Part print with two shaded views. Sizes in mm from the minimum x, y, z corner. Give positions to 0.01 mm unless a question says otherwise; leave off trailing zeros. Order: outer loops, then holes, each group sorted by start corner. A loop starts at its lowest first (then second) coordinate and runs counter-clockwise, first axis right, second up. Notation, with made-up numbers: (81, -36) -> (94, -36) arc R6 ccw to (94, -31) -> close; hole circle Ø4 at (38, -13). An arc over 180 degrees is marked (long way). Write item = value, one per line. Start each with the question number.
Item 1: Flat gauge pins, fed straight in: P1, Ø3, axis at x = 11.5, z = 11.5, coming from the +Y side; P2, Ø12, axis at x = 176, z = 55.5, coming from the +Y side. Where does each tip first touch, or does it go through?
Item 2: Band-saw the part on B-B on x = 111.5. Write the cut outline in (y, z).
Item 3: Band-saw the part on D-D on x = 76.5. Write the cut outline in (y, z), plus the area to 3 significant figures.
Item 4: Drill centre lines: line 1 along X through (y, z) = (3.75, 11.5); line 2 along Z through (x, y) = (211.5, 7); line 3 along X through (y, z) = (1, 12.5). Where is each one in solid material? Low to high.
Item 5: Band-saw the part on A-A on z = 86.5. Write the cut outline in (x, y).
Item 6: Band-saw the part on C-C on z = 18.5. Write the cut outline in (x, y), plus the area to 3 significant figures.
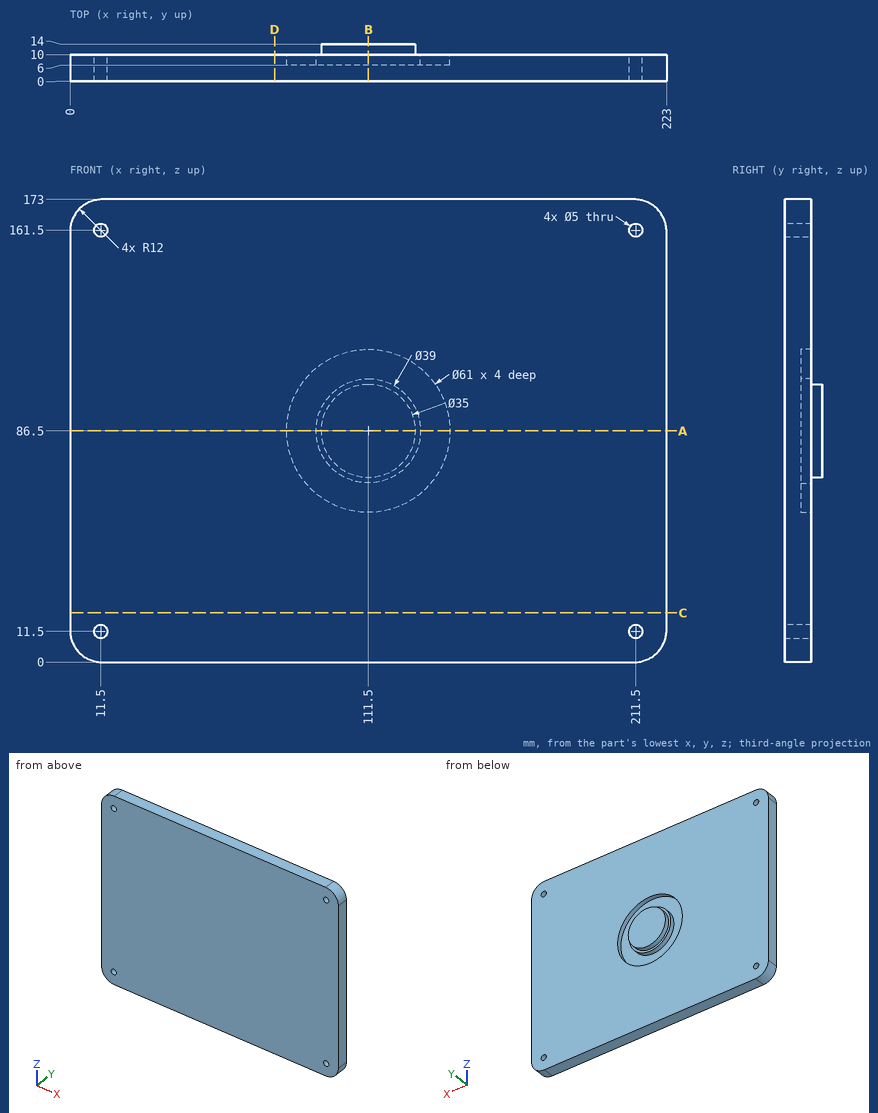
Values found:
q1.P1 = through
q1.P2 = 10
q2.outline = (0, 0) -> (10, 0) -> (10, 56) -> (6, 56) -> (6, 67) -> (10, 67) -> (10, 69) -> (14, 69) -> (14, 104) -> (10, 104) -> (10, 106) -> (6, 106) -> (6, 117) -> (10, 117) -> (10, 173) -> (0, 173) -> close
q3.outline = (0, 0) -> (10, 0) -> (10, 173) -> (0, 173) -> close
q3.area = 1,730 mm^2
q4.line_1 = 0.01 to 9, 14 to 209, 214 to 222.99
q4.line_2 = 0.01 to 9, 14 to 159, 164 to 172.99
q4.line_3 = 0 to 9.21, 13.79 to 209.21, 213.79 to 223
q5.outline = (0, 0) -> (223, 0) -> (223, 10) -> (142, 10) -> (142, 6) -> (131, 6) -> (131, 10) -> (129, 10) -> (129, 14) -> (94, 14) -> (94, 10) -> (92, 10) -> (92, 6) -> (81, 6) -> (81, 10) -> (0, 10) -> close
q6.outline = (0, 0) -> (223, 0) -> (223, 10) -> (0, 10) -> close
q6.area = 2,230 mm^2
